```python
from build123d import *

# Parameters (mm, degrees)
F0_W     = 110
F0_H     = 70
F1_DEPTH = 75
F3_DEPTH = 75.001
F4_W     = 65
F4_H     = 50
F5_DEPTH = 25
F6_W     = 10
F6_H     = 30
F7_DEPTH = 75.001
F8_W     = 70
F8_H     = 75
F9_DEPTH = 10


with BuildPart() as f1:
    # F0 (on Top) → F1 (new body)
    with BuildSketch(Plane.XY):
        with Locations((55, 35)):
            Rectangle(F0_W, F0_H)
    extrude(amount=F1_DEPTH)

    # F2 (on face) → F3 (cut, through all)
    with BuildSketch(Plane.XY.offset(75)):
        Polygon((0, 0), (90, 0), (90, 30), (75, 30), (75, 35), (47.5, 35), (47.5, 20), (0, 20), align=None)
    extrude(amount=-F3_DEPTH, mode=Mode.SUBTRACT)

    # F4 (on face) → F5 (cut)
    with BuildSketch(Plane.XY.offset(75)):
        with Locations((57.5, 45)):
            Rectangle(F4_W, F4_H)
    extrude(amount=-F5_DEPTH, mode=Mode.SUBTRACT)

    # F6 (on face) → F7 (cut, through all)
    with BuildSketch(Plane.XY.offset(75)):
        with Locations((95, 15)):
            Rectangle(F6_W, F6_H)
    extrude(amount=-F7_DEPTH, mode=Mode.SUBTRACT)

    # F8 (on face) → F9 (join)
    with BuildSketch(Plane.YZ.offset(110)):
        with Locations((35, 37.5)):
            Rectangle(F8_W, F8_H)
    extrude(amount=F9_DEPTH)


solid = f1.part
```
Check sheet for the modelled part. Datum: model origin and axes. Units: mm. A direction names the side the tool comes from. Round coordinates to 2 decimals unless told otherwise and drop trailing zeros. Loops run counter-clockwise (first coordinate to the right, second up) from the corner with the lowest first, then second, coordinate; pieces in that order, holes last. Notation, with made-up numbers: (-18.5, 21) -> (1.5, 21) arc R15 ccw to (1.5, 26) -> close; hole circle Ø9 at (-18, 39.25). An arc over 180 degrees is marked (long way). Answer in a Markdown table with one row per item.
Q1. Sectioned sample at A-A on y = 26.5. Enter the section's corners in (x, z), then the cut area to 3 significant figures.
Data:
| item | result |
|---|---|
| outline | (0, 0) -> (47.5, 0) -> (47.5, 50) -> (25, 50) -> (25, 75) -> (0, 75) -> close; (100, 0) -> (120, 0) -> (120, 75) -> (100, 75) -> close |
| area | 4,500 mm^2 |
Q2. Sectioned sample at C-C on z = 36. Enter the section's corners in (x, y).
Data:
| item | result |
|---|---|
| outline | (0, 20) -> (47.5, 20) -> (47.5, 35) -> (75, 35) -> (75, 30) -> (100, 30) -> (100, 0) -> (120, 0) -> (120, 70) -> (0, 70) -> close |
Q3. Go/stop test with flat-tipped pins: P1, Ø1, axis at y = 13.5, z = 39, coming from the -X side; P2, Ø4, axis at x = 46, z = 42, coming from the -Y side; P3, Ø3, axis at x = 50.5, z = 17, coming from the -Y side. Record where each tip stops, or that it passes through.
Data:
| item | result |
|---|---|
| P1 | stops at x = 100 |
| P2 | stops at y = 20 |
| P3 | stops at y = 35 |
Q4. Sectioned sample at D-D on x = 12. Enter the section's corners in (y, z).
Data:
| item | result |
|---|---|
| outline | (20, 0) -> (70, 0) -> (70, 75) -> (20, 75) -> close |
Q5. Thickness scan on L1, parallel to X at y = 25, z = 9.5; L2, parallel to X at y = 62.5, z = 56; L3, parallel to Y at x = 90.5, z = 29. Record the ranges inside material, lowest first.
Data:
| item | result |
|---|---|
| L1 | x = 0 to 47.5, 100 to 120 |
| L2 | x = 0 to 25, 90 to 120 |
| L3 | y = 30 to 70 |
Q6. Set-up check for faces 1 (the face through (120, 35, 38)), 2 (the face through (90, 50, 63)), 3 (the face through (47.5, 28, 25)), 4 (the face through (24, 20, 30)), 5 (the face through (12, 45, 75)): record each of +Z, -Z, +X, -X, +Y, -Y from which the full face is reachable in a straight line by a thin tool's end or side.
Data:
| item | result |
|---|---|
| face 1 | +Z, -Z, +X, +Y, -Y |
| face 2 | +Z, +Y, -Y |
| face 3 | +Z, -Z, -Y |
| face 4 | +Z, -Z, -X, -Y |
| face 5 | +Z, +X, -X, +Y, -Y |
Q7. Sectioned sample at B-B on z = 64.5. Enter the section's corners in (x, y).
Data:
| item | result |
|---|---|
| outline | (0, 20) -> (25, 20) -> (25, 70) -> (0, 70) -> close; (90, 30) -> (100, 30) -> (100, 0) -> (120, 0) -> (120, 70) -> (90, 70) -> close |
